```python
from build123d import *

# Parameters (mm, degrees)
SKETCH1_W           = 31.75
SKETCH1_H           = 31.75
SKETCH1_R           = 2.38125
BOSS_EXTRUDE1_DEPTH = 6.35
SKETCH2_W           = 66.675
SKETCH2_H           = 6.35
BOSS_EXTRUDE2_DEPTH = 19.05
SKETCH3_R           = 1.5875
CUT_EXTRUDE1_DEPTH  = 63.217039467
FILLET1_R           = 2.54


with BuildPart() as part:
    # Sketch1 → Boss-Extrude1 (new body)
    with BuildSketch(Plane.XY):
        Rectangle(SKETCH1_W, SKETCH1_H)
        with Locations((-11.1125, -3.175)):
            Circle(SKETCH1_R, mode=Mode.SUBTRACT)
        with Locations((-11.1125, 9.525)):
            Circle(SKETCH1_R, mode=Mode.SUBTRACT)
        with Locations((11.1125, 9.525)):
            Circle(SKETCH1_R, mode=Mode.SUBTRACT)
        with Locations((11.1125, -3.175)):
            Circle(SKETCH1_R, mode=Mode.SUBTRACT)
    extrude(amount=BOSS_EXTRUDE1_DEPTH)

    # Sketch2 → Boss-Extrude2 (add)
    with BuildSketch(Plane.XY.offset(6.35)):
        with Locations((-17.4625, -12.7)):
            Rectangle(SKETCH2_W, SKETCH2_H)
    extrude(amount=BOSS_EXTRUDE2_DEPTH)

    # Sketch3 → Cut-Extrude1 (cut, through all)
    with BuildSketch(Plane(origin=(0, -9.525, 0), x_dir=(1, 0, 0), z_dir=(0, 1, 0))):
        with Locations(Location((9.525, -18.542, 0), (0, 0, 270))):
            Circle(SKETCH3_R)
        with Locations(Location((-42.8625, -18.542, 0), (0, 0, 270))):
            Circle(SKETCH3_R)
    extrude(amount=-CUT_EXTRUDE1_DEPTH, mode=Mode.SUBTRACT)

    # Fillet1
    fillet1_edges = [part.edges().sort_by_distance(p)[0] for p in [
        (-50.8, -12.7, 6.35),
        (-50.8, -12.7, 25.4),
        (15.875, -12.7, 25.4),
        (-15.875, 15.875, 3.175),
        (15.875, 15.875, 3.175),
    ]]
    fillet(fillet1_edges, radius=FILLET1_R)


solid = part.part
```
Design review of the part built by this model. Coordinates are the model's own, in mm. A direction names the side the tool comes from. Coordinates: 2 decimals unless noted, no trailing zeros. Order: outer loops, then holes, each group sorted by start corner. A loop starts at its lowest first (then second) coordinate and runs counter-clockwise, first axis right, second up.
1) Mouldability with a two-part tool opening along Z and no side actions: class faces 4 (the cylindrical face through (8.56, -12.66, 17.28)), 5 (the cylindrical face through (-9.83, 11.53, 3.13)), 6 (the cylindrical face through (-50.076, -12.656, 7.114)), 7 (the cylindrical face through (-44.412, -12.656, 18.198)) as +Z half, -Z half, draft (parallel to the pull), parting line (faces both ways), or undercut.
2) Take a section at D-D, the plane z = 13. Give the boundary of the cut face in (x, y) (3 decimals).
3) Wall thickness on line 1 along X through (y, z) = (-3, 3) (3 decimals); line 2 along Z through (x, y) = (9, 11); line 3 along X through (y, z) = (7.5, 6) (3 decimals): over which ranges is each line inside the solid? List them lowest first.
4) Take a section at A-A, the plane x = -11. Give the boundary of the cut face in (y, z) (3 decimals), and give its area (3 significant figures).
5) For faces 1 (the cylindrical face through (15.111, -12.656, 24.676)), 2 (the flat face through (0, 3, 6.35)), 3 (the flat face through (-32, -13, 6.35)), list the 3-axis set-ups (+Z, -Z, +X, -X, +Y, -Y) from which the entire face can be reached by the end or side of a thin tool; tool diameter is ignored.
6) Take a section at B-B, the plane z = 19.5. Give the boundary of the cut face in (x, y) (3 decimals), and give its area (3 significant figures).
7) Take a section at C-C, the plane y = 11. Give the boundary of the cut face in (x, z) (3 decimals), and give its area (3 significant figures).
8) Clearance check with flat-ended pins moving along their axes: pin 1 (5 mm diameter, centred on x = 9.525, z = 18.542, fed in from -Y) (3 decimals); pin 2 (15 mm diameter, centred on x = -18.5, z = 13, fed in from +Y) (3 decimals); pin 3 (5 mm diameter, centred on x = -26, y = -14, fed in from -Z); pin 4 (3 mm diameter, centred on x = 11.11, y = 9.52, fed in from +Z). State where each tip first meets the part, or that it passes through.
Returned:
1. face 4: undercut
1. face 5: draft
1. face 6: -Z half
1. face 7: undercut
2. outline: (-50.8, -15.875) - (15.875, -15.875) - (15.875, -9.525) - (-50.8, -9.525) - close
3. line 1: x = -15.875 to -13.487, -8.738 to 8.738, 13.487 to 15.875
3. line 2: z = 0 to 6.35
3. line 3: x = -15.875 to -12.365, -9.86 to 9.86, 12.365 to 15.875
4. outline: (-15.875, 0) - (-5.554, 0) - (-5.554, 6.35) - (-9.525, 6.35) - (-9.525, 25.4) - (-15.875, 25.4) - close; (-0.796, 0) - (7.146, 0) - (7.146, 6.35) - (-0.796, 6.35) - close; (11.904, 0) - (15.875, 0) - (15.875, 6.35) - (11.904, 6.35) - close
4. area: 262 mm2
5. face 1: +Z, +X, +Y, -Y
5. face 2: +Z, +X, -X, +Y
5. face 3: -Z, -X, +Y, -Y
6. outline: (-50.8, -15.875) - (-44.128, -15.875) - (-44.128, -9.525) - (-50.8, -9.525) - close; (-41.597, -15.875) - (8.259, -15.875) - (8.259, -9.525) - (-41.597, -9.525) - close; (10.791, -15.875) - (15.875, -15.875) - (15.875, -9.525) - (10.791, -9.525) - close
6. area: 391 mm2
7. outline: (-15.875, 0) - (-12.982, 0) - (-12.982, 6.35) - (-15.875, 6.35) - close; (-9.243, 0) - (9.243, 0) - (9.243, 6.35) - (-9.243, 6.35) - close; (12.982, 0) - (15.875, 0) - (15.875, 6.35) - (12.982, 6.35) - close
7. area: 154 mm2
8. pin 1: stops at y = -15.875
8. pin 2: stops at y = 15.225
8. pin 3: stops at z = 6.35
8. pin 4: passes through
